Input: part model. Units: mm. Frame: model coordinates. A direction names the side the tool comes from. Round coordinates to 2 decimals unless told otherwise and drop trailing zeros. Loops run counter-clockwise (first coordinate to the right, second up) from the corner with the lowest first, then second, coordinate; pieces in that order, holes last. Notation, with made-up numbers: (19.5, -25.75) -> (44.5, -25.75) arc R16 cw to (44.5, 3.25) -> close; hole circle Ø4 at (-14.5, 65.25). An arc over 180 degrees is marked (long way). Answer as a JSON object with one key per item and string values. Group by question number.
Item 1: Section query C-C on x = 0. Return loops of the section in (y, z), and give its area (3 significant figures).
Item 2: Section query A-A on z = 0. Return loops of the section in (x, y), and give its area (3 significant figures).
Item 3: Pin query (flat end, axial travel): pin 1 (2.5 mm diameter, centred on x = -1.5, y = -23.5, fed in from +Z); pin 2 (3 mm diameter, centred on x = -4.5, y = -25.5, fed in from -Z); pin 3 (3 mm diameter, centred on y = -20, z = -5, fed in from -X). Return the tip coordinate at first contact, or that it passes through.
Item 4: Draft query along X for faces 1 (the cylindrical face through (-4.76, -28.59, -3.65)), 2 (the cylindrical face through (0.29, -52.93, 2.23)), 3 (the flat face through (0, -25, 4)). Return one class per face: released by +X, released by -X, zero draft, split by the parting line, or undercut.
Item 5: Material intervals for line 1 (Y direction, x = 1.5, z = 5.75); line 2 (Z direction, x = 0, y = -54.25); line 3 (Z direction, x = 0, y = -38), sorted ascending. Write a range as [from, to].
Item 6: Section query B-B on y = -23.5. Return loops of the section in (x, z).
Item 7: Set-up query: faces 4 (the cylindrical face through (-0.596, -23.664, -2.685)), 5 (the flat face through (3, 0, -1)), 6 (the flat face through (0, -20, 5)), 7 (the flat face through (0, -30, -5)). Return all of +Z, -Z, +X, -X, +Y, -Y with unobstructed straight access to the full face (end or side cutting, diameter ignored); none if empty.
Item 8: Section query D-D on z = 4.75. Return loops of the section in (x, y), and give its area (3 significant figures).
from build123d import *

# Parameters (mm, degrees)
F0_R          = 6
F1_DEPTH      = 58
F2_R          = 2.75
F3_DEPTH      = 48
F4_W          = 10
F4_H          = 2
F5_DEPTH      = 6.001
F5_DEPTH_BACK = 6.001
F7_D          = 4.5
F7_DEPTH      = 10
F7_TIP        = 1.3519363928


with BuildPart() as f1:
    # F0 (on Front) → F1 (new body)
    with BuildSketch(Plane.XZ):
        Circle(F0_R)
    extrude(amount=F1_DEPTH)

    # F2 (on Front) → F3 (cut)
    with BuildSketch(Plane.XZ):
        Circle(F2_R)
    extrude(amount=F3_DEPTH, mode=Mode.SUBTRACT)

    # F4 (on Right) → F5 (cut, two sides)
    with BuildSketch(Plane.YZ) as f5_sk:
        with Locations((-25, -5)):
            Rectangle(F4_W, F4_H)
        with Locations((-25, 5)):
            Rectangle(F4_W, F4_H)
    extrude(amount=F5_DEPTH, mode=Mode.SUBTRACT)
    extrude(f5_sk.sketch, amount=-F5_DEPTH_BACK, mode=Mode.SUBTRACT)

    # F7
    with Locations(Plane.XZ.offset(58)):
        with Locations((0, 0)):
            Hole(F7_D / 2, depth=F7_DEPTH)
            with Locations((0, 0, -(F7_DEPTH + F7_TIP / 2))):  # 118° drill point
                Cone(0, F7_D / 2, F7_TIP, mode=Mode.SUBTRACT)


solid = f1.part
Solved:
{
 "1": {"outline": "(-58, -6) -> (-30, -6) -> (-30, -4) -> (-20, -4) -> (-20, -6) -> (0, -6) -> (0, -2.75) -> (-48, -2.75) -> (-48, -2.25) -> (-58, -2.25) -> close; (-58, 2.25) -> (-48, 2.25) -> (-48, 2.75) -> (0, 2.75) -> (0, 6) -> (-20, 6) -> (-20, 4) -> (-30, 4) -> (-30, 6) -> (-58, 6) -> close", "area": "347 mm²"},
 "2": {"outline": "(-6, -58) -> (-2.25, -58) -> (-2.25, -48) -> (-2.75, -48) -> (-2.75, 0) -> (-6, 0) -> close; (2.25, -58) -> (6, -58) -> (6, 0) -> (2.75, 0) -> (2.75, -48) -> (2.25, -48) -> close", "area": "387 mm²"},
 "3": {"pin 1": "z = 4", "pin 2": "z = -4", "pin 3": "x = -4.87"},
 "4": {"face 1": "split by the parting line", "face 2": "undercut", "face 3": "zero draft"},
 "5": {"line 1": "[-58, -30], [-20, 0]", "line 2": "[-6, -2.25], [2.25, 6]", "line 3": "[-6, -2.75], [2.75, 6]"},
 "6": {"outline": "(-4.47, -4) -> (4.47, -4) arc R6 ccw to (4.47, 4) -> (-4.47, 4) arc R6 ccw to start; hole circle Ø5.5 at (0, 0)"},
 "7": {"face 4": "+Y", "face 5": "+Z, -Z, +X, -X, +Y", "face 6": "+Z, +X, -X", "face 7": "-Z, +X, -X"},
 "8": {"outline": "(-3.67, -58) -> (3.67, -58) -> (3.67, -30) -> (-3.67, -30) -> close; (-3.67, -20) -> (3.67, -20) -> (3.67, 0) -> (-3.67, 0) -> close", "area": "352 mm²"}
}
